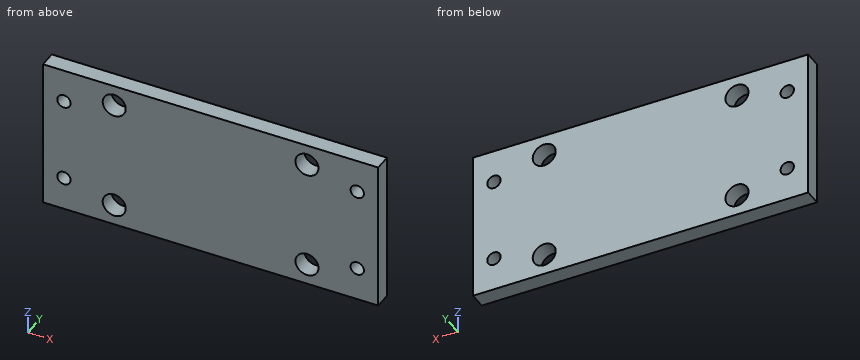
from build123d import *

# Parameters (mm, degrees)
SKETCH_1_R      = 2.75
SKETCH_1_R_2    = 1.6
EXTRUDE_1_DEPTH = 4


with BuildPart() as part:
    # 草图1 → 凸台-拉伸1 (new body)
    with BuildSketch(Plane(origin=(0, 0, 0), x_dir=(1, 0, 0), z_dir=(0, 1, 0))):
        Polygon((-34.919077445, 32.481158859), (33.080922555, 32.481158859), (33.080922555, -3.518841141), (-34.919077445, -3.518841141), (-46.919077445, -3.518841141), (-46.919077445, 32.481158859), align=None)
        with Locations((-29.919077445, 27.481158859)):
            Circle(SKETCH_1_R, mode=Mode.SUBTRACT)
        with Locations((16.080922555, 27.481158859)):
            Circle(SKETCH_1_R, mode=Mode.SUBTRACT)
        with Locations((-29.919077445, 1.481158859)):
            Circle(SKETCH_1_R, mode=Mode.SUBTRACT)
        with Locations((16.080922555, 1.481158859)):
            Circle(SKETCH_1_R, mode=Mode.SUBTRACT)
        with Locations((-41.919077445, 24.481158859)):
            Circle(SKETCH_1_R_2, mode=Mode.SUBTRACT)
        with Locations((28.080922555, 24.481158859)):
            Circle(SKETCH_1_R_2, mode=Mode.SUBTRACT)
        with Locations((-41.919077445, 4.481158859)):
            Circle(SKETCH_1_R_2, mode=Mode.SUBTRACT)
        with Locations((28.080922555, 4.481158859)):
            Circle(SKETCH_1_R_2, mode=Mode.SUBTRACT)
    extrude(amount=EXTRUDE_1_DEPTH)


solid = part.part
Geometry check sheet. Reference: the model listing, model coordinates, mm. Coordinates: 2 decimals unless noted, no trailing zeros. Order: outer loops, then holes, each group sorted by start corner. A loop starts at its lowest first (then second) coordinate and runs counter-clockwise, first axis right, second up. Notation, with made-up numbers: (-27, 36) - (13, 36) arc R16 ccw to (13, 66) - close; hole circle Ø2 at (-36, -39). An arc over 180 degrees is marked (long way). Answer in a Markdown table with one row per item. Add a question column.
1) Material ranges on line 1 along X through (y, z) = (0.9, -29); line 2 along X through (y, z) = (0.85, -3.5); line 3 along Z through (x, y) = (-28, 2.3), recorded low to high. Write a range as [from, to].
2) Cross-section at B-B, the plane y = 0.6. State how many separate pieces and enclosed holes the cut face has, then the cut area to 3 significant figures.
3) Gauge pin test, flat ends, axial feed: P1, Ø7, axis at x = 16.08, z = -1.48, coming from the +Y side; P2, Ø3, axis at x = 28.08, z = -4.48, coming from the +Y side. Record the tip position at first contact, or that the pin passes through.
4) Cross-section at A-A, the plane z = -29. Record the cut outline in (x, y), then the cut area to 3 significant figures.
Check result:
| question | item | result |
|---|---|---|
| 1 | line 1 | x = [-46.92, -32.21], [-27.63, 13.79], [18.37, 33.08] |
| 1 | line 2 | x = [-46.92, -43.18], [-40.66, -31.79], [-28.05, 14.21], [17.95, 26.82], [29.34, 33.08] |
| 1 | line 3 | z = [-32.48, -29.45], [-25.51, -3.45], [0.49, 3.52] |
| 2 | separate pieces | 1 |
| 2 | enclosed holes | 8 |
| 2 | area | 2,750 mm² |
| 3 | P1 | stops at y = 4 |
| 3 | P2 | passes through |
| 4 | outline | (-46.92, 0) - (-32.21, 0) - (-32.21, 4) - (-46.92, 4) - close; (-27.63, 0) - (13.79, 0) - (13.79, 4) - (-27.63, 4) - close; (18.37, 0) - (33.08, 0) - (33.08, 4) - (18.37, 4) - close |
| 4 | area | 283 mm² |
